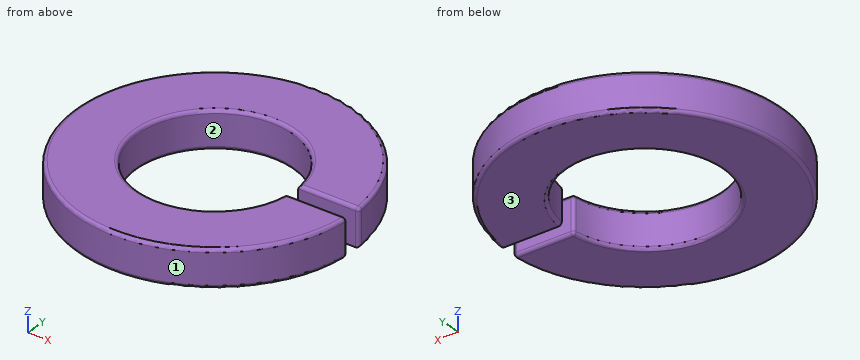
```python
from build123d import *

# Parameters (mm, degrees)
RESSALTO_EXTRUS_O1_DEPTH = 2.3
FILETE1_R                = 0.2


with BuildPart() as part:
    # Esboço1 → Ressalto-extrusão1 (new body)
    with BuildSketch(Plane.XY):
        with BuildLine():
            Line((4.73869444, 0.5), (8.485281374, 0.5))
            ThreePointArc((8.485281374, 0.5), (-8.5, 0), (8.485281374, -0.5))
            Line((8.485281374, -0.5), (4.73869444, -0.5))
            ThreePointArc((4.73869444, -0.5), (-4.765, 0), (4.73869444, 0.5))
        make_face()
    extrude(amount=RESSALTO_EXTRUS_O1_DEPTH)

    # Filete1
    filete1_edges = [part.edges().sort_by_distance(p)[0] for p in [
        (-8.5, 0, 2.3),
        (6.611987907, -0.5, 2.3),
        (-4.765, 0, 2.3),
        (6.611987907, -0.5, 0),
        (-8.5, 0, 0),
        (-4.765, 0, 0),
        (6.611987907, 0.5, 2.3),
        (4.73869444, -0.5, 1.15),
        (8.485281374, -0.5, 1.15),
        (8.485281374, 0.5, 1.15),
    ]]
    fillet(filete1_edges, radius=FILETE1_R)


solid = part.part
```
Model file for the job. Use its own axes, mm. Face numbers are marked on the shaded views. Give positions to 0.01 mm unless a question says otherwise; leave off trailing zeros. Write each loop counter-clockwise with the first axis right and the second up, starting at its lowest first coordinate (ties: lowest second). Pieces come first, ordered by that corner, then holes. Notation, with made-up numbers: (64, 41.5) - (120, 41.5) arc R23 ccw to (120, 64.5) - close; hole circle Ø11 at (35, 14). An arc over 180 degrees is marked (long way). One line per question, with ' | ' between items. Start each with the question number.
(1) Wall check: line 1 along Y through (x, z) = (0, 1.1) (3 decimals); line 2 along Y through (x, z) = (6, 0.85); line 3 along X through (y, z) = (1, 0.75). Give the ranges that are in metal, low to high. Write a range as from..to.
(2) Two-plate mould, pull along Y, no slides. Class the marked faces 1, 2 and 3: +Y half, -Y half, draft (parallel to the pull), parting line (faces both ways), or undercut.
(3) Pin check, flat tips, straight feed: P1, Ø0.6, axis at x = 5.5, z = 1, coming from the -Y side; P2, Ø4, axis at x = -1.5, y = -1.5, coming from the +Z side. Stop position of each tip, or through.
(4) Slice it at A-A on z = 1.2. Write the cut outline in (x, y) (3 decimals).
Results below:
1) line 1: -8.5..-4.765, 4.765..8.5 | line 2: -6.02..-0.5, 0.5..6.02 | line 3: -8.44..-4.66, 4.66..8.44
2) face 1: parting line | face 2: undercut | face 3: draft
3) P1: y = -6.72 | P2: through
4) outline: (4.717, -0.672) arc R4.765 cw (long way) to (4.739, 0.5) - (8.27, 0.5) arc R0.2 ccw to (8.47, 0.717) arc R8.5 ccw (long way) to (8.47, -0.717) arc R0.2 ccw to (8.27, -0.5) - (4.915, -0.5) arc R0.2 ccw to start
